For this review, take the finished solid that the model builds, in its own axes (mm). A direction names the side the tool comes from. Coordinates: 2 decimals unless noted, no trailing zeros. Loops run counter-clockwise (first coordinate to the right, second up) from the corner with the lowest first, then second, coordinate; pieces in that order, holes last. Notation, with made-up numbers: (87.5, -39) - (135.5, -39) arc R21 ccw to (135.5, -5) - close; hole circle Ø5 at (80, 83.25). An arc over 180 degrees is marked (long way). One line per item, written item: value. Start each with the question number.
1. The part is to be moulded in two halves that separate along Y. For faces 3 (the face through (0.03, -6.55, 1.97)), 4 (the face through (25.865, -10.724, 5.24)), 5 (the face through (0, -12, 6)), 6 (the face through (-0.943, -4.247, 1.972)), say which applies: released by +Y, released by -Y, zero draft, split by the parting line, or undercut.
2. To check wall thickness, follow line 1 (Z direction, x = -6, y = -4); line 2 (Y direction, x = 0, z = 5); line 3 (Y direction, x = -4, z = 2.35). State the ranges of each line that lie inside material, in increasing order. Write a range as from..to.
3. Take a section at A-A, the plane x = 0. State the section outline as (y, z) points, and give its area (3 significant figures).
4. For faces 1 (the face through (6, 0, 0)), 2 (the face through (-2.17, -9.76, 4.99)), list the 3-axis set-ups (+Z, -Z, +X, -X, +Y, -Y) from which the entire face can be reached by the end or side of a thin tool; tool diameter is ignored.
5. Take a section at C-C, the plane z = 0.75. State the section outline as (x, y) points.
6. Insertion check: pin 1 (1.2 mm diameter, centred on x = 0, y = 7.3, fed in from -Z); pin 2 (6 mm diameter, centred on x = -3, y = -5.5, fed in from +Z). Each pin has a flat end and moves straight along its axis. Give the tip position at first contact, or say it passes through.
```python
from build123d import *

# Parameters (mm, degrees)
CYLINDER003_R     = 0.75
CYLINDER003_DEPTH = 10
ARRAY_COUNT       = 4
CYLINDER002_R     = 4.35
CYLINDER002_DEPTH = 10
CYLINDER001_R     = 10
CYLINDER001_DEPTH = 10
TORUS_R           = 1.5
CYLINDER_R        = 28
CYLINDER_DEPTH    = 6


with BuildPart() as array:
    # Cylinder003 → Cylinder003 (new body)
    with BuildSketch(Plane(origin=(7.3, 0, -5), x_dir=(1, 0, 0), z_dir=(0, 0, 1))):
        Circle(CYLINDER003_R)
    extrude(amount=CYLINDER003_DEPTH)

    # Array: Array ×4 about axis
    array_axis = Axis((0, 0, 0), (0, 0, 1))


with BuildPart() as array_1:
    add(array.part)
    for i in range(1, ARRAY_COUNT):
        add(array.part.rotate(array_axis, i * 360 / ARRAY_COUNT))


with BuildPart() as cylinder002:
    # Cylinder002 → Cylinder002 (new body)
    with BuildSketch(Plane.XY.offset(-4)):
        Circle(CYLINDER002_R)
    extrude(amount=CYLINDER002_DEPTH)


with BuildPart() as corona_serve:
    # Cylinder001 → Cylinder001 (new body)
    with BuildSketch(Plane.XY.offset(4)):
        Circle(CYLINDER001_R)
    extrude(amount=CYLINDER001_DEPTH)


with BuildPart() as torus:
    # Torus → Torus (revolve)
    with BuildSketch(Plane(origin=(0, 0, 3), x_dir=(1, 0, 0), z_dir=(0, -1, 0))):
        with Locations((28, 0)):
            Circle(TORUS_R)
    revolve(axis=Axis((0, 0, 3), (0, 0, 1)))


with BuildPart() as cut003:
    # Cylinder → Cylinder (new body)
    with BuildSketch(Plane.XY):
        Circle(CYLINDER_R)
    extrude(amount=CYLINDER_DEPTH)

    # Cut: cut Torus
    add(torus.part, mode=Mode.SUBTRACT)

    # Cut001: cut corona_serve
    add(corona_serve.part, mode=Mode.SUBTRACT)

    # Cut002: cut Cylinder002
    add(cylinder002.part, mode=Mode.SUBTRACT)

    # Cut003: cut Array
    add(array_1.part, mode=Mode.SUBTRACT)


solid = cut003.part
```
Solutions:
1. face 3: undercut
1. face 4: split by the parting line
1. face 5: zero draft
1. face 6: undercut
2. line 1: 0..4
2. line 2: -28..-10, 10..28
2. line 3: -26.35..-1.71, 1.71..26.35
3. outline: (-28, 0) - (-8.05, 0) - (-8.05, 4) - (-10, 4) - (-10, 6) - (-28, 6) - (-28, 4.5) arc R1.5 cw to (-28, 1.5) - close; (-6.55, 0) - (-4.35, 0) - (-4.35, 4) - (-6.55, 4) - close; (4.35, 0) - (6.55, 0) - (6.55, 4) - (4.35, 4) - close; (8.05, 0) - (28, 0) - (28, 1.5) arc R1.5 cw to (28, 4.5) - (28, 6) - (10, 6) - (10, 4) - (8.05, 4) - close
3. area: 242 mm2
4. face 1: -Z, +X, -X, +Y, -Y
4. face 2: +Z
5. outline: circle Ø56 at (0, 0); hole circle Ø1.5 at (-7.3, 0); hole circle Ø8.7 at (0, 0); hole circle Ø1.5 at (0, -7.3); hole circle Ø1.5 at (0, 7.3); hole circle Ø1.5 at (7.3, 0)
6. pin 1: through
6. pin 2: z = 4
